from build123d import *
from build123d.topology import SkipClean

# Parameters (mm, degrees)
SKETCH10_R              = 10
BOSS_EXTRUDE1_DEPTH     = 5
CUT_EXTRUDE3_DEPTH      = 45
CUT_EXTRUDE3_DEPTH_BACK = 20
CUT_EXTRUDE5_DEPTH      = 5
BOSS_EXTRUDE2_DEPTH     = 5
SKETCH14_R              = 1
BOSS_EXTRUDE3_DEPTH     = 3
SKETCH15_R              = 1
BOSS_EXTRUDE4_DEPTH     = 3


with BuildPart() as part:
    # Sketch1 → Revolve1 (revolve)
    with BuildSketch(Plane.XY):
        with BuildLine():
            Line((20.9, 0), (23.871591838, 0))
            Line((23.871591838, 0), (23.871591838, 4))
            Line((23.871591838, 4), (22.9, 4.236662843))
            Line((22.9, 4.236662843), (22.9, 11.404308102))
            ThreePointArc((22.9, 11.404308102), (23.83692213, 15.63049072), (26.472123903, 19.064752533))
            Line((26.472123903, 19.064752533), (26.988320528, 19.497892931))
            ThreePointArc((26.988320528, 19.497892931), (29.623522302, 22.932154745), (30.560444431, 27.158337362))
            Line((30.560444431, 27.158337362), (30.560444431, 50))
            ThreePointArc((30.560444431, 50), (29.388871556, 52.828427125), (26.560444431, 54))
            Line((26.560444431, 54), (2.764914955, 54))
            Line((2.764914955, 54), (2.764914955, 15))
            Line((2.764914955, 15), (19.9, 15))
            ThreePointArc((19.9, 15), (20.607106781, 14.707106781), (20.9, 14))
            Line((20.9, 14), (20.9, 0))
        make_face()
    revolve(axis=Axis((2.764914955, 7.821821657, 0), (0, 1, 0)))

    # Sketch10 → Boss-Extrude1 (add)
    with SkipClean():  # the faces are left unmerged after this step: merging them gives an invalid solid
        with BuildSketch(Plane.XY.offset(27.795529476)):
            with Locations((3.346345887, 38.658337362)):
                Circle(SKETCH10_R)
        extrude(amount=-BOSS_EXTRUDE1_DEPTH)

    # Sketch11 → Cut-Extrude3 (cut, two sides: drawn at the far end of the back side and taken through both)
    with SkipClean():  # the faces are left unmerged after this step: merging them gives an invalid solid
        with BuildSketch(Plane(origin=(0, 17, 0), x_dir=(1, 0, 0), z_dir=(0, 1, 0)).offset(-CUT_EXTRUDE3_DEPTH_BACK)):
            with BuildLine():
                Line((-14.735085045, 0), (20.264914955, 0))
                ThreePointArc((20.264914955, 0), (2.764914955, 17.5), (-14.735085045, 0))
            make_face()
        extrude(amount=CUT_EXTRUDE3_DEPTH + CUT_EXTRUDE3_DEPTH_BACK, mode=Mode.SUBTRACT)

    # Sketch9 → Cut-Extrude5 (cut)
    with SkipClean():  # the faces are left unmerged after this step: merging them gives an invalid solid
        with BuildSketch(Plane(origin=(0, 54, 0), x_dir=(1, 0, 0), z_dir=(0, 1, 0))):
            with BuildLine():
                Line((-25.235085045, 0), (30.764914955, 0))
                ThreePointArc((30.764914955, 0), (2.764914955, 28), (-25.235085045, 0))
            make_face()
        extrude(amount=-CUT_EXTRUDE5_DEPTH, mode=Mode.SUBTRACT)

    # Sketch13 → Boss-Extrude2 (add)
    with SkipClean():  # the faces are left unmerged after this step: merging them gives an invalid solid
        with BuildSketch(Plane(origin=(0, 0, 0), x_dir=(-1, 0, 0), z_dir=(0, 0, -1))):
            with BuildLine():
                Line((17.53061452, 53), (21.53061452, 53))
                ThreePointArc((21.53061452, 53), (21.884167911, 52.853553391), (22.03061452, 52.5))
                Line((22.03061452, 52.5), (22.03061452, 50.5))
                ThreePointArc((22.03061452, 50.5), (21.884167911, 50.146446609), (21.53061452, 50))
                Line((21.53061452, 50), (17.53061452, 50))
                ThreePointArc((17.53061452, 50), (17.17706113, 50.146446609), (17.03061452, 50.5))
                Line((17.03061452, 50.5), (17.03061452, 52.5))
                ThreePointArc((17.03061452, 52.5), (17.17706113, 52.853553391), (17.53061452, 53))
            make_face()
            with BuildLine():
                Line((-27.060444431, 52.75), (-23.060444431, 52.75))
                ThreePointArc((-23.060444431, 52.75), (-22.706891041, 52.603553391), (-22.560444431, 52.25))
                Line((-22.560444431, 52.25), (-22.560444431, 50.25))
                ThreePointArc((-22.560444431, 50.25), (-22.706891041, 49.896446609), (-23.060444431, 49.75))
                Line((-23.060444431, 49.75), (-27.060444431, 49.75))
                ThreePointArc((-27.060444431, 49.75), (-27.413997822, 49.896446609), (-27.560444431, 50.25))
                Line((-27.560444431, 50.25), (-27.560444431, 52.25))
                ThreePointArc((-27.560444431, 52.25), (-27.413997822, 52.603553391), (-27.060444431, 52.75))
            make_face()
        extrude(amount=BOSS_EXTRUDE2_DEPTH)

    # Sketch14 → Boss-Extrude3 (add)
    with SkipClean():  # the faces are left unmerged after this step: merging them gives an invalid solid
        with BuildSketch(Plane.ZY.offset(-22.560444431)):
            with Locations(Location((-3, 51.25, 0), (0, 0, 270))):
                Circle(SKETCH14_R)
        extrude(amount=BOSS_EXTRUDE3_DEPTH)

    # Sketch15 → Boss-Extrude4 (add)
    with SkipClean():  # the faces are left unmerged after this step: merging them gives an invalid solid
        with BuildSketch(Plane(origin=(-17.03061452, 0, 0), x_dir=(0, 0, -1), z_dir=(1, 0, 0))):
            with Locations(Location((3, 51.5, 0), (0, 0, 270))):
                Circle(SKETCH15_R)
        extrude(amount=BOSS_EXTRUDE4_DEPTH)


solid = part.part
The listing builds one solid part. Answer for the finished solid, in the listing's coordinates (mm). A direction names the side the tool comes from. Coordinates: 2 decimals unless noted, no trailing zeros. Write each loop counter-clockwise with the first axis right and the second up, starting at its lowest first coordinate (ties: lowest second). Pieces come first, ordered by that corner, then holes. Notation, with made-up numbers: (-23, 48) - (18, 48) arc R17 cw to (18, 76) - close; hole circle Ø6 at (-21.75, 16.5). An arc over 180 degrees is marked (long way). Answer as CSV lines item,"result".
1. A tool of negligible diameter and unlimited length cuts with its end or side. For faces 4 (the cylindrical face through (-6.65, 38.87, 27.17)), 5 (the flat face through (25, 49.75, -2)), 6 (the cylindrical face through (-1.811, 2.028, 20.605)), 7 (the flat face through (-17.031, 51.5, -4.4)), 8 (the flat face through (-20, 50, -2)), from which of +Z, -Z, +X, -X, +Y, -Y can it reach the whole face along a straight path? Write none if from no direction.
Computed values:
face 4,"+Z, -X"
face 5,"-Z, +X, -X"
face 6,"-Y"
face 7,"-Z"
face 8,"-Z, -X"
2. Find section A-A (y = 36). Give the vertices of the cut face in (x, z), plus the area to 3 significant figures.
Computed values:
outline,"(-6.29, 26.28) arc R27.8 ccw (long way) to (12.99, 25.85) - (12.99, 27.8) - (-6.29, 27.8) - close; hole (-14.74, 0) arc R17.5 ccw to (20.26, 0) - close"
area,"1,960 mm²"
3. Straight lines are drawn through the part: line 1 (X direction, y = 10.25, z = 0); line 2 (X direction, y = 3.25, z = 0); line 3 (X direction, y = 32.5, z = 1). For each, find the intervals that lie inside material, in ascending order. Write a range as [from, to].
Computed values:
line 1,"x = [-17.37, -15.37], [20.9, 22.9]"
line 2,"x = [-18.34, -15.37], [20.9, 23.87]"
line 3,"x = [-25.01, 30.54]"
4. Given P1, Ø2, axis at x = 23, y = 39.5, coming from the +Z side; P2, Ø8, axis at x = -15.5, y = 29.5, coming from the +Z side; P3, Ø2, axis at y = 51.5, z = -2.5, coming from the +X side; P4, Ø19, axis at x = -1.5, z = 10, coming from the -Y side, each flat-ended and moving along its own axis, determine where each tip first touches the part or whether it passes through.
Computed values:
P1,"stops at z = 20.06"
P2,"stops at z = 23.86"
P3,"stops at x = 27.56"
P4,"stops at y = 0"
5. Determine the mould class of faces 1 (the flat face through (-14.031, 52, -3)), 2 (the flat face through (-20, 52, -5)), 3 (the cylindrical face through (-15.552, 50.546, -3.3)) for opening direction Z: +Z half, -Z half, draft (parallel to the pull), parting line (faces both ways), or undercut.
Computed values:
face 1,"draft"
face 2,"-Z half"
face 3,"undercut"
